Design review of the part built by this model. Coordinates are the model's own, in mm. A direction names the side the tool comes from. Give positions to 0.01 mm unless a question says otherwise; leave off trailing zeros. Order: outer loops, then holes, each group sorted by start corner. A loop starts at its lowest first (then second) coordinate and runs counter-clockwise, first axis right, second up. Notation, with made-up numbers: M 80.25,-26 L 116.25,-26 A22 ccw 116.25,-7 Z; hole C 14,87.25 d6. An arc over 180 degrees is marked long. Answer as a JSON object with one key per item and string values.
from build123d import *

# Parameters (mm, degrees)
SKETCH_2_R          = 2.6
CUT_EXTRUDE_1_DEPTH = 49.512884886


with BuildPart() as part:
    # 草图1 → 旋转1 (revolve)
    with BuildSketch(Plane.XY, mode=Mode.PRIVATE) as revolve_1_sk:
        Polygon((0, 0), (27.5, 0), (27.5, 4), (9, 4), (9, 10), (5.95, 10), (5.95, 21), (5.45, 21), (5.45, 22), (5.95, 22), (5.95, 23), (4, 23), (4, 33), (0, 33), (0, 23.5), align=None)
    revolve(revolve_1_sk.sketch.rotate(Axis((0, 23.5, 0), (0, -1, 0)), 90), axis=Axis((0, 23.5, 0), (0, -1, 0)))

    # 草图2 → 切除-拉伸1 (cut, through all)
    with BuildSketch(Plane(origin=(0, 4, 0), x_dir=(1, 0, 0), z_dir=(0, 1, 0))):
        with Locations(Location((22.5, 0, 0), (0, 0, 270))):
            Circle(SKETCH_2_R)
        with Locations(Location((11.25, -19.485571585, 0), (0, 0, 270))):
            Circle(SKETCH_2_R)
        with Locations(Location((-11.25, -19.485571585, 0), (0, 0, 270))):
            Circle(SKETCH_2_R)
        with Locations(Location((-22.5, 0, 0), (0, 0, 270))):
            Circle(SKETCH_2_R)
        with Locations(Location((-11.25, 19.485571585, 0), (0, 0, 270))):
            Circle(SKETCH_2_R)
        with Locations(Location((11.25, 19.485571585, 0), (0, 0, 270))):
            Circle(SKETCH_2_R)
    extrude(amount=-CUT_EXTRUDE_1_DEPTH, mode=Mode.SUBTRACT)


solid = part.part
(1) To check wall thickness, follow L1, parallel to Y at x = 10, z = 13.5; L2, parallel to Z at x = 22, y = 2; L3, parallel to Y at x = 6, z = 6. State the ranges of each line that lie inside material, in increasing order. Write a range as from..to.
Checked values:
{"L1": "y = 0..4", "L2": "z = -16.5..-2.55, 2.55..16.5", "L3": "y = 0..10"}
(2) We need section A-A (z = 0). Count the separate pieces of the cut face and the enclosed holes in it, plus the area to 3 significant figures.
Checked values:
{"separate pieces": "3", "enclosed holes": "0", "area": "520 mm^2"}
(3) We need section D-D (y = 7). Write out the cut boundary in (x, z), plus the area to 3 significant figures.
Checked values:
{"outline": "C 0,0 d18", "area": "254 mm^2"}
(4) Insertion check: pin 1 (6 mm diameter, centred on x = 11.25, z = 19.49, fed in from +Y); pin 2 (6 mm diameter, centred on y = 23.5, z = -5, fed in from +X); pin 3 (5 mm diameter, centred on x = 9.5, y = 15.5, fed in from +Z); pin 4 (10 mm diameter, centred on y = 22.5, z = 4, fed in from -X). Each pin has a flat end and moves straight along its axis. Give the tip position at first contact, or say it passes through.
Checked values:
{"pin 1": "stops at y = 4", "pin 2": "stops at x = 5.59", "pin 3": "passes through", "pin 4": "stops at x = -5.95"}
(5) We need section C-C (x = -22.5). Write out the cut boundary in (y, z), plus the area to 3 significant figures.
Checked values:
{"outline": "M 0,-15.81 L 4,-15.81 L 4,-2.6 L 0,-2.6 Z; M 0,2.6 L 4,2.6 L 4,15.81 L 0,15.81 Z", "area": "106 mm^2"}
(6) We need section B-B (x = -11.25). Write out the cut boundary in (y, z).
Checked values:
{"outline": "M 0,-25.09 L 4,-25.09 L 4,-22.09 L 0,-22.09 Z; M 0,-16.89 L 4,-16.89 L 4,16.89 L 0,16.89 Z; M 0,22.09 L 4,22.09 L 4,25.09 L 0,25.09 Z"}
(7) Tool access review of faces 1 (the cylindrical face through (-12.246, 2.028, 21.887)), 2 (the cylindrical face through (-6.083, 7.042, -6.633)): name each direction out of +Z, -Z, +X, -X, +Y, -Y from which nothing blocks a thin tool from reaching the whole face with its end or side.
Checked values:
{"face 1": "+Y, -Y", "face 2": "+Y"}
